Print and shaded views of the part. All mm, measured from the part's lowest x, y and z. Round coordinates to 2 decimals unless told otherwise and drop trailing zeros. Write each loop counter-clockwise with the first axis right and the second up, starting at its lowest first coordinate (ties: lowest second). Pieces come first, ordered by that corner, then holes. Notation, with made-up numbers: M 76,57.25 L 116,57.25 A22 ccw 116,69.25 Z; hole C 65.25,14.25 d11. An arc over 180 degrees is marked long. Write item = value, one per line. Start each with the question number.
Q1. Band-saw the part on B-B on y = 18.25. Write the cut outline in (x, z), plus the area to 3 significant figures.
Q2. Band-saw the part on D-D on y = 29.5. Write the cut outline in (x, z).
Q3. Band-saw the part on C-C on z = 0.7. State how many separate pieces and enclosed holes the cut face has, plus the area to 3 significant figures.
Q4. Drop flat-ended pins along their axis: P1, Ø4.5, axis at x = 40, y = 28.25, coming from the +Z side (3 decimals); P2, Ø6, axis at x = 91, y = 8.25, coming from the +Z side. Give the stop position or say it passes through.
Q5. Band-saw the part on A-A on x = 60. Write the cut outline in (y, z).
Q6. Probe L1, parallel to X at y = 22, z = 0.6; L2, parallel to X at y = 27, z = 1; L3, parallel to Y at x = 23, z = 1.3. List the from-to ranges inside material, lowest first.
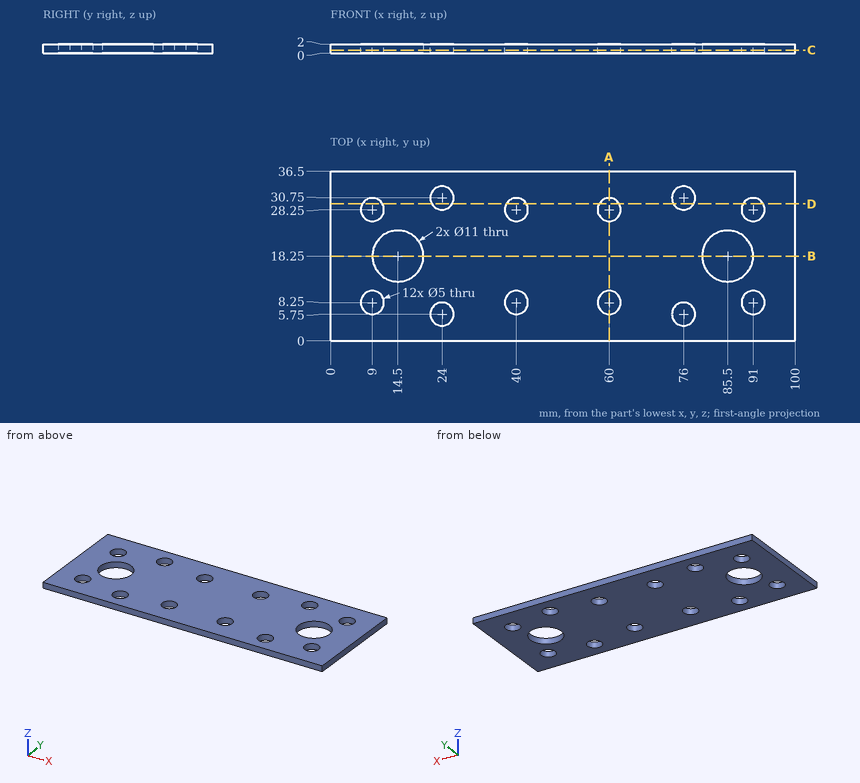
Conclusion:
q1.outline = M 0,0 L 9,0 L 9,2 L 0,2 Z; M 20,0 L 80,0 L 80,2 L 20,2 Z; M 91,0 L 100,0 L 100,2 L 91,2 Z
q1.area = 156 mm^2
q2.outline = M 0,0 L 6.83,0 L 6.83,2 L 0,2 Z; M 11.17,0 L 21.83,0 L 21.83,2 L 11.17,2 Z; M 26.17,0 L 37.83,0 L 37.83,2 L 26.17,2 Z; M 42.17,0 L 57.83,0 L 57.83,2 L 42.17,2 Z; M 62.17,0 L 73.83,0 L 73.83,2 L 62.17,2 Z; M 78.17,0 L 88.83,0 L 88.83,2 L 78.17,2 Z; M 93.17,0 L 100,0 L 100,2 L 93.17,2 Z
q3.separate_pieces = 1
q3.enclosed_holes = 14
q3.area = 3,220 mm^2
q4.P1 = through
q4.P2 = 2
q5.outline = M 0,0 L 5.75,0 L 5.75,2 L 0,2 Z; M 10.75,0 L 25.75,0 L 25.75,2 L 10.75,2 Z; M 30.75,0 L 36.5,0 L 36.5,2 L 30.75,2 Z
q6.L1 = 0 to 10.48, 18.52 to 81.48, 89.52 to 100
q6.L2 = 0 to 6.83, 11.17 to 37.83, 42.17 to 57.83, 62.17 to 88.83, 93.17 to 100
q6.L3 = 0 to 3.46, 8.04 to 28.46, 33.04 to 36.5
